For this review, take the finished solid that the model builds, in its own axes (mm). A direction names the side the tool comes from. Coordinates: 2 decimals unless noted, no trailing zeros. Loops run counter-clockwise (first coordinate to the right, second up) from the corner with the lowest first, then second, coordinate; pieces in that order, holes last. Notation, with made-up numbers: (83.25, 16.5) - (140.25, 16.5) arc R16 cw to (140.25, 23.5) - close; hole circle Ø7 at (18.5, 70.25). An arc over 180 degrees is marked (long way). One line per item, written item: value. Start each with the question number.
1. For faces 5 (the face through (-22.05, -46.56, 16.42)), 6 (the face through (30.82, 49.91, 8.95)), 7 (the face through (0, 42, 16)), list the 3-axis set-ups (+Z, -Z, +X, -X, +Y, -Y) from which the entire face can be reached by the end or side of a thin tool; tool diameter is ignored.
2. To check wall thickness, follow line 1 (Z direction, x = -18.5, y = -31); line 2 (X direction, y = 7.5, z = 2.25); line 3 (X direction, y = -37, z = 5). State the ranges of each line that lie inside material, in increasing order. Write a range as from..to.
3. Take a section at A-A, the plane z = 16.35. State the section outline as (x, y) points.
4. Take a section at B-B, the plane z = 7.75. Count the separate pieces of the cut face and the enclosed holes in it, and give its area (3 significant figures).
5. Insertion check: pin 1 (0.8 mm diameter, centred on y = 50, z = 6, fed in from +X); pin 2 (1.5 mm diameter, centred on y = 19.5, z = 22.5, fed in from -X); pin 3 (2 mm diameter, centred on x = -12.5, z = 15, fed in from -Y). Each pin has a flat end and moves straight along its axis. Give the tip position at first contact, or say it passes through.
6. The part is to be moulded in two halves that separate along X. For faces 1 (the face through (3, 12, 4)), 2 (the face through (-0.4, 49, 23.5)), 3 (the face through (-31.822, 2, 8)), 4 (the face through (35, -1, 10)), say which applies: released by +X, released by -X, zero draft, split by the parting line, or undercut.
```python
from build123d import *

# Parameters (mm, degrees)
SKETCH016_W        = 70
SKETCH016_H        = 102
PAD007_DEPTH       = 26
SKETCH017_W        = 60
SKETCH017_H        = 92
POCKET011_DEPTH    = 6.5
FILLET010_R        = 3
SKETCH018_W        = 59
SKETCH018_H        = 84
POCKET012_DEPTH    = 7.5
POCKET013_DEPTH    = 9
POCKET014_DEPTH    = 8
POCKET015_DEPTH    = 8
CHAMFER007_SIZE2   = 5
CHAMFER007_SIZE    = 4
FILLET011_R        = 5
FILLET012_R        = 3
POCKET015_FACE20_W = 2
POCKET015_FACE20_H = 8
POCKET016_DEPTH    = 0.356442
FILLET013_R        = 3.5


with BuildPart() as part:
    # Sketch016 → Pad007 (new body)
    with BuildSketch(Plane.XY):
        Rectangle(SKETCH016_W, SKETCH016_H)
    extrude(amount=PAD007_DEPTH)

    # Sketch017 (on Face6 of Pad007) → Pocket011 (cut)
    with BuildSketch(Plane.XY.offset(26)):
        Rectangle(SKETCH017_W, SKETCH017_H)
    extrude(amount=-POCKET011_DEPTH, mode=Mode.SUBTRACT)

    # Fillet010
    fillet010_edges = [part.edges().sort_by_distance(p)[0] for p in [
        (30, 46, 22.75),
        (-30, 46, 22.75),
        (-30, -46, 22.75),
        (30, -46, 22.75),
    ]]
    fillet(fillet010_edges, radius=FILLET010_R)

    # Sketch018 (on Face11 of Pocket011) → Pocket012 (cut)
    with BuildSketch(Plane.XY.offset(19.5)):
        Rectangle(SKETCH018_W, SKETCH018_H)
    extrude(amount=-POCKET012_DEPTH, mode=Mode.SUBTRACT)

    # Sketch019 (on Face13 of Pocket012) → Pocket013 (cut)
    with BuildSketch(Plane.XZ.offset(51)):
        with BuildLine():
            ThreePointArc((-18.9, 19.5), (-22.05, 16.35), (-18.9, 13.2))
            Line((-18.9, 13.2), (-12.6, 13.2))
            ThreePointArc((-12.6, 13.2), (-9.45, 16.35), (-12.6, 19.5))
            Line((-12.6, 19.5), (-18.9, 19.5))
        make_face()
    extrude(amount=-POCKET013_DEPTH, mode=Mode.SUBTRACT)

    # Sketch020 (on DatumPlane) → Pocket014 (cut)
    with BuildSketch(Plane(origin=(0, 0, 2), x_dir=(1, 0, 0), z_dir=(0, 0, -1))):
        with BuildLine():
            Line((-31.821779, 47), (-31.821779, 51))
            Line((-31.821779, 51), (-0.178221, 51))
            Line((-0.178221, 51), (-0.178221, 47))
            add(Edge.make_bspline(
                [(-0.178221, 47), (-27, -46.775214), (-0.178221, -49)],
                knots=[0, 0, 0, 1, 1, 1], degree=2))
            Line((-0.178221, -49), (-0.178221, -51))
            Line((-0.178221, -51), (-31.821779, -51))
            Line((-31.821779, -51), (-31.821779, -49))
            add(Edge.make_bspline(
                [(-31.821779, 47), (-5, -46.775214), (-31.821779, -49)],
                knots=[0, 0, 0, 1, 1, 1], degree=2))
        make_face()
        with BuildLine():
            Line((31.821779, 47), (31.821779, 51))
            Line((31.821779, 51), (0.178221, 51))
            Line((0.178221, 51), (0.178221, 47))
            add(Edge.make_bspline(
                [(0.178221, 47), (27, -46.775214), (0.178221, -49)],
                knots=[0, 0, 0, 1, 1, 1], degree=2))
            Line((0.178221, -49), (0.178221, -51))
            Line((0.178221, -51), (31.821779, -51))
            Line((31.821779, -51), (31.821779, -49))
            add(Edge.make_bspline(
                [(31.821779, 47), (5, -46.775214), (31.821779, -49)],
                knots=[0, 0, 0, 1, 1, 1], degree=2))
        make_face()
    extrude(amount=-POCKET014_DEPTH, mode=Mode.SUBTRACT)

    # Sketch021 (on DatumPlane) → Pocket015 (cut)
    with BuildSketch(Plane.XY.offset(12)):
        with BuildLine():
            add(Edge.make_bspline(
                [(0, -41.6971), (-22.282957, 30.899597), (0, 64.842011), (22.282957, 30.899597), (0, -41.6971)],
                knots=[0, 0, 0, 0, 0.5, 1, 1, 1, 1], degree=3))
        make_face()
        with BuildLine():
            Line((-31.821779, 48.104515), (-31.821779, -45.461681))
            add(Edge.make_bspline(
                [(-31.821779, 48.104515), (-7.061375, 47.212971), (-31.821779, -45.461681)],
                knots=[0, 0, 0, 1, 1, 1], degree=2))
        make_face()
    extrude(amount=-POCKET015_DEPTH, mode=Mode.SUBTRACT)

    # Chamfer007
    chamfer007_edges = [part.edges().sort_by_distance(p)[0] for p in [
        (0, 51, 26),
        (-35, 0, 26),
        (35, 0, 26),
        (0, -51, 26),
    ]]
    chamfer007_side = part.faces().sort_by_distance((-31.237093, 0, 26))[0]
    chamfer(chamfer007_edges, length=CHAMFER007_SIZE, length2=CHAMFER007_SIZE2, reference=chamfer007_side)

    # Fillet011
    fillet011_edges = [part.edges().sort_by_distance(p)[0] for p in [
        (-33, -49, 23.5),
        (-33, 49, 23.5),
        (33, -49, 23.5),
        (33, 49, 23.5),
    ]]
    fillet(fillet011_edges, radius=FILLET011_R)

    # Fillet012
    fillet012_edges = [part.edges().sort_by_distance(p)[0] for p in [
        (35, 51, 9.834634),
        (-35, 51, 9.834634),
        (-35, -51, 9.834634),
        (35, -51, 9.834634),
    ]]
    fillet(fillet012_edges, radius=FILLET012_R)

    # Pocket015 Face20 → Pocket016 (cut)
    with BuildSketch(Plane(origin=(-0.178221, 50, 6), x_dir=(0, 1, 0), z_dir=(-1, 0, 0))):
        Rectangle(POCKET015_FACE20_W, POCKET015_FACE20_H)
    extrude(amount=-POCKET016_DEPTH, mode=Mode.SUBTRACT)

    # Fillet013
    fillet013_edges = [part.edges().sort_by_distance(p)[0] for p in [
        (-31.821779, 50, 10),
        (31.821779, 50, 10),
        (-31.821779, 50, 2),
        (31.821779, 50, 2),
    ]]
    fillet(fillet013_edges, radius=FILLET013_R)


solid = part.part
```
Solutions:
1. face 5: -Y
1. face 6: +Y
1. face 7: +Z
2. line 1: 0..2, 10..12
2. line 2: -35..-19.61, -12.39..12.39, 19.61..35
2. line 3: -35..-31.82, -29.62..-29.04, -2.96..-1.42, 1.42..2.96, 29.04..35
3. outline: (-35, -48) arc R3 ccw to (-32, -51) - (-22.05, -51) - (-22.05, -42) - (-29.5, -42) - (-29.5, 42) - (29.5, 42) - (29.5, -42) - (-9.45, -42) - (-9.45, -51) - (32, -51) arc R3 ccw to (35, -48) - (35, 48) arc R3 ccw to (32, 51) - (-32, 51) arc R3 ccw to (-35, 48) - close
4. separate pieces: 3
4. enclosed holes: 2
4. area: 1,780 mm2
5. pin 1: x = 34.54
5. pin 2: x = -34.4
5. pin 3: y = 42
6. face 1: undercut
6. face 2: zero draft
6. face 3: undercut
6. face 4: released by +X
